Autodesk Inventor part; units mm, degrees
ref_plane "Work Plane1" through (7, 3.5, 17.0635) normal (0, 1, 0) x (1, 0, 0)
ref_plane "Work Plane3" through (0, 3.0314, 24) normal (1, 0, 0) x (0, 0, -1)
ref_plane "YZ Plane" through (0, 0, 0) normal (1, 0, 0) x (0, 1, 0)
sketch "Sketch1" plane through (0, 0, 0) normal (0, 0, 1) x (1, 0, 0)
  line L0 (0, 14) -> (0, 11)
  line L1 (0, 14) -> (15, 14)
  line L2 (15, 14) -> (15, 0)
  circle A0 centre (0, 7) radius 4
  line L3 (0, 3) -> (0, 0) construction
  line L4 (0, 0) -> (15, 0)
  line L5 (0, 11) -> (0, 3) construction
  line L6 (0.5, 0) -> (-0.5, 0)
  line L7 (-0.5, 0) -> (-0.5, 3.0314)
  line L8 (-0.5, 3.0314) -> (0.5, 3.0314)
  line L9 (0.5, 3.0314) -> (0.5, 0)
  line L10 (-0.5, 0) -> (-7, 0)
  line L11 (-7, 0) -> (-7, 14)
  line L12 (-7, 14) -> (0, 14)
  line L13 (-4, 10.1012) -> (-4, 3.4286) construction
  point P0 (0, 3.0314)
  dimension "d0" = 8
  dimension "d1" = 15
  dimension "d2" = 14
  dimension "d79" = 1
  dimension "d80" = 3
  dimension "d81" = 3
extrude "Extrusion1" add sketch "Sketch1" along normal blind 24 contours L1 L2 L4 L9 A0 L0 | L0 A0 L7 L10 L11 L12
sketch "Sketch2" plane through (15, 0, 0) normal (1, 0, 0) x (0, 0, -1)
  line L0 (-24, 0) -> (-24, 14)
  line L1 (0, 0) -> (0, 14)
  point P0 (-19, 7)
  point P1 (-5, 7)
  point P2 (-24, 7)
  dimension "d5" = 5
  dimension "d6" = 5
  dimension "d7" = 14
hole "Hole1" at (15, 7, 19) at (15, 7, 5) direction (-1, 0, 0) diameter 4 depth 8
sketch "Sketch4" plane through (0, 14, 0) normal (0, 1, 0) x (1, 0, 0)
  circle A0 centre (9.5, -5) radius 3.5
  circle A1 centre (9.5, -19) radius 3.5
  line L0 (15, -24) -> (-7, -24)
  line L1 (15, 0) -> (0, 0)
  line L2 (-0.5, 0) -> (0.5, 0)
  line L3 (-0.5, -24) -> (0.5, -24)
  line L4 (4, -24) -> (4, 0)
  line L5 (4, -24) -> (4, 0)
  line L6 (4, -24) -> (4, 0)
  line L7 (15, 0) -> (15, -24)
  line L8 (0.5, 0) -> (0.5, -24)
  line L9 (-0.5, 0) -> (-0.5, -24)
  point P0 (4, -24)
  point P1 (0, -24)
  dimension "d18" = 7
  dimension "d19" = 7
  dimension "d20" = 14
  dimension "d21" = 5
  dimension "d22" = 5
  dimension "d42" = 5.5
  dimension "d43" = 5.5
extrude "Extrusion2" add sketch "Sketch4" along normal blind 1 contours A0 | A1
sketch "Sketch3" plane through (2, 15, 0) normal (0, 1, 0) x (1, 0, 0)
  circle A0 centre (7.5, -5) radius 3.5
  circle A1 centre (7.5, -19) radius 3.5
hole "Hole2" at (9.5, 15, 19) at (9.5, 15, 5) direction (0, -1, 0) diameter 4 depth 7
sketch "Sketch5" plane through (15, 0, 0) normal (1, 0, 0) x (0, 0, -1)
  line L0 (-17.0635, 7.5) -> (-6.9365, 7.5)
  line L1 (-6.9365, 7.5) -> (-6.9365, 6.5)
  line L2 (-6.9365, 6.5) -> (-17.0635, 6.5)
  line L3 (-17.0635, 6.5) -> (-17.0635, 7.5)
  circle A0 centre (-5, 7) radius 2
  circle A1 centre (-19, 7) radius 2
  point P0 (0, 0)
  point P1 (-6.9365, 7)
  point P2 (-17.0635, 6.5)
  dimension "d35" = 1
extrude "Extrusion3" cut sketch "Sketch5" against normal blind 8 contours L0 A0 L2 A1
sketch "Sketch7" plane through (0, 14, 0) normal (0, 1, 0) x (1, 0, 0)
  circle A0 centre (9.5, -5) radius 2
  circle A1 centre (9.5, -19) radius 2
  point P0 (0, 0)
  point P1 (9.5, -12)
  dimension "d44" = 7
  dimension "d45" = 7
hole "Hole3" at (9.5, 14, 12) direction (0, -1, 0) diameter 3.4 end through all countersink diameter 6.3 countersink angle 90
chamfer "Chamfer3" distance 0.5 angle 45 2 edges at (15, 7, 21) (15, 7, 3)
ref_plane "Work Plane1" through (7, 3.5, 17.0635) normal (0, 1, 0) x (1, 0, 0)
sketch "Sketch10" plane through (7, 3.5, 17.0635) normal (0, 1, 0) x (1, 0, 0)
  circle A0 centre (2.5, 5.0635) radius 1.7
  line L0 (-0.25, 3.4758) -> (-0.25, 6.6512)
  line L1 (-0.25, 6.6512) -> (2.5, 8.2389)
  line L2 (2.5, 8.2389) -> (5.25, 6.6512)
  line L3 (5.25, 6.6512) -> (5.25, 3.4758)
  line L4 (5.25, 3.4758) -> (2.5, 1.8881)
  line L5 (2.5, 1.8881) -> (-0.25, 3.4758)
  point P0 (-7, 17.0635)
  dimension "d75" = 5.5
extrude "Extrusion6" cut sketch "Sketch10" against normal blind 10
sketch "Sketch12" plane through (-0.5, 0, 0) normal (1, 0, 0) x (0, 0, -1)
  circle A0 centre (-12, -3.25) radius 1.7
  circle A1 centre (-12, -3.25) radius 5.25
  line L0 (0, 0) -> (-8.616, -7.2639)
  line L1 (-24, 0) -> (-15.384, -7.2639)
  circle A2 centre (-12, -3.25) radius 3.25
  line L2 (0, 0) -> (-24, 0)
  point P0 (-12, 0)
  dimension "d82" = 3.4
  dimension "d84" = 2
  dimension "d95" = 6.5
extrude "Extrusion7" add sketch "Sketch12" against normal blind 5.5 contours A0 | A2 | A1 L2 | L1 L2 A1 | A1 L2 L0 picked at (-14.5812, -7.0055)
ref_plane "Work Plane3" through (0, 3.0314, 24) normal (1, 0, 0) x (0, 0, -1)
mirror "Mirror1" about plane through (0, 3.0314, 24) normal (1, 0, 0) of "Extrusion7"
fillet "Fillet1" radius 7 1 edges at (-7, 14, 12)
sketch "Sketch14" plane through (-6, 3.5, 13.5877) normal (1, 0, 0) x (0, 0, -1)
  arc A0 (-1.7963, -10.7639) -> (4.9717, -10.7639) centre (1.5877, -6.75) ccw
  line L0 (0, -9.5) -> (-1.5877, -6.75)
  line L1 (-1.5877, -6.75) -> (0, -4)
  line L2 (0, -4) -> (3.1754, -4)
  line L3 (3.1754, -4) -> (4.7631, -6.75)
  line L4 (4.7631, -6.75) -> (3.1754, -9.5)
  line L5 (3.1754, -9.5) -> (0, -9.5)
  point P0 (13.5877, -3.5)
  dimension "d96" = 5.5
extrude "Extrusion8" cut sketch "Sketch14" along normal blind 2.5
sketch "Sketch13" plane through (6, 0, 0) normal (-1, 0, 0) x (0, 0, 1)
  arc A0 (8.616, -7.2639) -> (15.384, -7.2639) centre (12, -3.25) ccw
  point P0 (0, 0)
hole "Hole4" at (6, -3.25, 12) direction (-1, 0, 0) diameter 3.4 end through all
sketch "Sketch15" plane through (0, 0, 24) normal (0, 0, 1) x (1, 0, 0)
  line L0 (6, 0) -> (15, 0)
  line L1 (15, 0) -> (15, 14)
  line L2 (14.5, 9) -> (14.5, 5)
  line L3 (15, 4.5) -> (15, 9.5)
  line L4 (6, 0) -> (15, 0)
  arc A0 (6, 0) -> (10.5, 1.125) centre (6, 9.5625) ccw
  line L5 (15, 0) -> (15, 14)
  arc A1 (15, 2.25) -> (10.5, 1.125) centre (15, -7.3125) ccw
  line L6 (15, 4.5) -> (15, 9.5)
  line L7 (15, 4.5) -> (15, 0)
  line L8 (15, 2.25) -> (10.6581, 2.25) construction
  point P0 (0, 0)
  point P1 (14.5, 6.5)
  point P2 (14.5, 7.5)
  point P3 (15, 7.5)
  point P4 (15, 6.5)
  point P5 (15, 2.25)
extrude "Extrusion9" cut sketch "Sketch15" against normal blind 28.75
chamfer "Chamfer5" distance 1 angle 45 13 edges at (0, 11, 24) (0, 11, 0) (-4.9497, 11.9497, 0) (-7, 3.5, 0) (7.5, 14, 0) (7.5, 14, 24) (-4.9497, 11.9497, 24) (-7, 3.5, 24) (-7, 0, 12) (8.3192, 0.2855, 0) (12.6808, 1.9645, 0) (12.6808, 1.9645, 24) (8.3192, 0.2855, 24)
chamfer "Chamfer6" distance 0.5 angle 45 2 edges at (6, 15, 19) (6, 15, 5)
chamfer "Chamfer7" distance 1.5 angle 45 1 edges at (6, -3.25, 13.7)
equation "\"d81\" = d80"
equation "\"d22\" = d21"
equation "\"d42\" = d43"
properties part number "XY Joiner"
The model under review builds one solid part; all positions refer to its coordinate system, in mm. A direction names the side the tool comes from. Coordinates: 2 decimals unless noted, no trailing zeros. Put each result on its own line as item: value.
1) Wall thickness on probe 1 along Z at (x, y) = (9.5, 12.5); probe 2 along Z at (x, y) = (9.5, 4.95); probe 3 along X at (y, z) = (7, 2.5): over which ranges is each line inside the solid? List them lowest first. Write a range as [from, to].
Computed:
probe 1: z = [0, 3], [7, 10.3], [13.7, 17], [21, 24]
probe 2: z = [0, 10.3], [13.7, 24]
probe 3: x = [-7, -4], [4, 15]
2) Clearance check with flat-ended pins moving along their axes: pin 1 Ø2.5 at (x, z) = (11.5, 11.5) entering from -Y; pin 2 Ø2 at (y, z) = (-3, 15) entering from +X; pin 3 Ø2.5 at (y, z) = (-3.25, 12) entering from -X; pin 4 Ø9.5 at (y, z) = (-5.5, 16) entering from -X. State where each tip first meets the part, or that it passes through.
Computed:
pin 1: stops at y = 1.85
pin 2: stops at x = 6
pin 3: passes through
pin 4: stops at x = -6
3) Add section B-B on y = 5.5. State how many separate pieces and enclosed holes the cut face has, then the cut area to 3 significant figures.
Computed:
separate pieces: 2
enclosed holes: 1
area: 295 mm2
4) Draft analysis for pull direction Z (two halves, no side actions). For faces 6 (the flat face through (7, 7, 24)), 7 (the flat face through (-3.212, -3.581, 4.248)), 8 (the cylindrical face through (-3.2, -8.5, 12.1)), 9 (the cylindrical face through (6.003, 14.246, 5.154)), state which applies: released by +Z, released by -Z, zero draft, split by the parting line, or undercut.
Computed:
face 6: released by +Z
face 7: released by -Z
face 8: split by the parting line
face 9: undercut
5) For faces 1 (the cylindrical face through (10.698, 5.106, 4.357)), 2 (the cylindrical face through (6.92, 14.246, 21.365)), 3 (the flat face through (6.75, 2, 12)), 4 (the flat face through (0.5, -1, 12)), 5 (the flat face through (-4.768, -4.644, 14.37)), list the 3-axis set-ups (+Z, -Z, +X, -X, +Y, -Y) from which the entire face can be reached by the end or side of a thin tool; tool diameter is ignored.
Computed:
face 1: +X
face 2: +Y
face 3: -Y
face 4: +Z, -Z, -Y
face 5: -X
